The model under review builds one solid part; all positions refer to its coordinate system, in mm. A direction names the side the tool comes from. Round coordinates to 2 decimals unless told otherwise and drop trailing zeros. Loops run counter-clockwise (first coordinate to the right, second up) from the corner with the lowest first, then second, coordinate; pieces in that order, holes last. Notation, with made-up numbers: M -11.75,38 L 27.25,38 A25 cw 27.25,52 Z; hole C -15,21.5 d5. An arc over 180 degrees is marked long. One line per question, with ' | ' between items.
Autodesk Inventor part; units mm, degrees
ref_plane "YZ Plane" through (0, 0, 0) normal (1, 0, 0) x (0, 1, 0)
ref_plane "XZ Plane" through (0, 0, 0) normal (0, 1, 0) x (-1, 0, 0)
ref_plane "XY Plane" through (0, 0, 0) normal (0, 0, 1) x (1, 0, 0)
sketch "スケッチ1" plane through (0, 0, 0) normal (0, 0, 1) x (1, 0, 0)
  line L0 (51, 14.4226) -> (51, -10.5774)
  line L1 (-51, -10.5774) -> (-51, 14.4226)
  circle A0 centre (-22.5, -0.0774) radius 1.6
  circle A1 centre (22.5, -0.0774) radius 1.6
  line L2 (-71, -27.5774) -> (71, -27.5774)
  line L3 (71, -27.5774) -> (71, -14.5774)
  line L4 (-53, -12.5774) -> (-69, -12.5774)
  line L5 (-71, -14.5774) -> (-71, -27.5774)
  arc A2 (-53, -12.5774) -> (-51, -10.5774) centre (-53, -10.5774) ccw
  line L6 (69, -12.5774) -> (53, -12.5774)
  arc A3 (51, -10.5774) -> (53, -12.5774) centre (53, -10.5774) ccw
  line L7 (-51, 14.4226) -> (51, 14.4226)
  arc A4 (-69, -12.5774) -> (-71, -14.5774) centre (-69, -14.5774) ccw
  arc A5 (71, -14.5774) -> (69, -12.5774) centre (69, -14.5774) ccw
  arc A6 (51, 14.4226) -> (-51, 14.4226) centre (0, -53.5774) ccw
  point P0 (0, 0)
  point P1 (0, -100)
  point P2 (71, -12.5774)
  point P3 (-71, -12.5774)
  point P4 (0, 31.4226)
  dimension "d5" = 51
  dimension "d8" = 3.2
  dimension "d10" = 3.2
  dimension "d28" = 45
  dimension "d31" = 28.5
  dimension "d35" = 142
  dimension "d36" = 15
  dimension "d38" = 2
  dimension "d39" = 2
  dimension "d42" = 20
  dimension "d47" = 100
  dimension "d48" = 51
  dimension "d55" = 102
  dimension "d56" = 42
  dimension "d57" = 2
  dimension "d58" = 2
  dimension "d73" = 27.5
  dimension "d75" = 27.5
  dimension "d76" = 17
  dimension "d86" = 20
extrude "押し出し1" add sketch "スケッチ1" along normal blind 38
sketch "スケッチ2" plane through (0, 0, 38) normal (0, 0, 1) x (1, 0, 0)
  line L0 (-39, 13.4226) -> (39, 13.4226)
  line L1 (46, 6.4226) -> (46, -10.5774)
  line L2 (44, -12.5774) -> (-44, -12.5774)
  line L3 (-46, -10.5774) -> (-46, 6.4226)
  arc A0 (-39, 13.4226) -> (-46, 6.4226) centre (-39, 6.4226) ccw
  arc A1 (46, 6.4226) -> (39, 13.4226) centre (39, 6.4226) ccw
  arc A2 (-46, -10.5774) -> (-44, -12.5774) centre (-44, -10.5774) ccw
  arc A3 (44, -12.5774) -> (46, -10.5774) centre (44, -10.5774) ccw
  circle A4 centre (22.5, -0.0774) radius 1.6
  point P0 (0, 0)
  point P1 (-46, 13.4226)
  point P2 (46, -12.5774)
  point P3 (46, 13.4226)
  point P4 (-46, -12.5774)
  dimension "d17" = 92
  dimension "d18" = 26
  dimension "d19" = 46
  dimension "d23" = 7
  dimension "d24" = 7
  dimension "d25" = 2
  dimension "d26" = 2
  dimension "d50" = 12.5
extrude "押し出し2" cut sketch "スケッチ2" against normal blind 33 contours L0 A1 L1 A3 L2 A2 L3 A0 | A4
sketch "スケッチ3" plane through (0, 0, 38) normal (0, 0, 1) x (1, 0, 0)
  line L0 (-39, 13.4226) -> (39, 13.4226)
  arc A0 (39, 13.4226) -> (-39, 13.4226) centre (0, -57.6274) ccw
  line L1 (-46, -10.5774) -> (-46, 6.4226)
  line L2 (44, -12.5774) -> (-44, -12.5774)
  line L3 (-39, 13.4226) -> (39, 13.4226)
  point P0 (0, 0)
  point P1 (0, 23.4226)
  dimension "d59" = 10
extrude "押し出し3" cut sketch "スケッチ3" against normal blind 40
sketch "スケッチ4" plane through (0, 0, 38) normal (0, 0, 1) x (1, 0, 0)
  line L0 (-31, -12.5774) -> (31, -12.5774)
  line L1 (31, -12.5774) -> (31, -20.5774)
  line L2 (29, -22.5774) -> (-29, -22.5774)
  line L3 (-31, -20.5774) -> (-31, -12.5774)
  line L4 (-46, -10.5774) -> (-46, 6.4226)
  line L5 (44, -12.5774) -> (-44, -12.5774)
  arc A0 (-31, -20.5774) -> (-29, -22.5774) centre (-29, -20.5774) ccw
  arc A1 (29, -22.5774) -> (31, -20.5774) centre (29, -20.5774) ccw
  point P0 (0, 0)
  point P1 (31, -22.5774)
  point P2 (-31, -22.5774)
  dimension "d66" = 62
  dimension "d67" = 10
  dimension "d68" = 15
  dimension "d69" = 10
  dimension "d72" = 2
extrude "押し出し4" cut sketch "スケッチ4" against normal blind 35
sketch "スケッチ5" plane through (-69, -12.5774, 0) normal (0, 1, 0) x (1, 0, 0)
  circle A0 centre (8, -18) radius 5.05
  line L0 (69, 0) -> (69, -40)
  circle A1 centre (130, -18) radius 5.05
  line L1 (18, 0) -> (18, -38)
  line L2 (16, -38) -> (0, -38)
  point P0 (-2, -38)
  dimension "d77" = 10.1
  dimension "d84" = 10
  dimension "d85" = 20
extrude "押し出し5" cut sketch "スケッチ5" against normal blind 5
sketch "スケッチ6" plane through (-61, -17.5774, 18) normal (0, 1, 0) x (1, 0, 0)
  line L0 (61, 18) -> (61, -20)
  line L1 (90, -20) -> (32, -20)
  circle A0 centre (0, 0) radius 2.6
  circle A1 centre (122, 0) radius 2.6
  line L2 (10, 18) -> (10, -20)
  line L3 (8, -20) -> (-8, -20)
  dimension "d81" = 5.2
  dimension "d87" = 10
  dimension "d88" = 20
extrude "押し出し6" cut sketch "スケッチ6" against normal blind 10
sketch "スケッチ7" plane through (-51, -10.5774, 0) normal (-1, 0, 0) x (0, 0, 1)
  line L0 (7, 19) -> (11, 19)
  line L1 (13, 17) -> (13, 5)
  line L2 (11, 3) -> (7, 3)
  line L3 (5, 5) -> (5, 17)
  arc A0 (7, 19) -> (5, 17) centre (7, 17) ccw
  arc A1 (5, 5) -> (7, 3) centre (7, 5) ccw
  arc A2 (11, 3) -> (13, 5) centre (11, 5) ccw
  arc A3 (13, 17) -> (11, 19) centre (11, 17) ccw
  line L4 (0, 25) -> (0, 0)
  point P0 (0, 10.5774)
  point P1 (13, 3)
  point P2 (13, 19)
  point P3 (5, 3)
  point P4 (38, -2)
  dimension "d89" = 8
  dimension "d90" = 16
  dimension "d91" = 2
  dimension "d94" = 5
  dimension "d95" = 5
extrude "押し出し7" cut sketch "スケッチ7" against normal blind 8
properties part number "jig"
1) For line 1 (Z direction, x = -61, y = -16); line 2 (Z direction, x = -46.5, y = 5); line 3 (X direction, y = -22.25, z = 18), list the stretches that pass through material, from the lowest coordinate up.
Output values:
line 1: z = 0 to 12.95, 23.05 to 38 | line 2: z = 0 to 5, 13 to 38 | line 3: x = -71 to -63.6, -58.4 to -30.1, 30.1 to 58.4, 63.6 to 71
2) Machinability: for faces 1 (the flat face through (-59, -12.577, 23)), 2 (the flat face through (0, -22.577, 21)), 3 (the flat face through (-1, -27.577, 19)), 4 (the flat face through (-59, -17.577, 20)), which of the approach directions +Z, -Z, +X, -X, +Y, -Y give a long, thin tool a straight path to every point of the face, cutting with its end or side? Answer none if there is none.
Output values:
face 1: +Z, -Z, -X, +Y | face 2: +Z | face 3: +Z, -Z, +X, -X, -Y | face 4: +Y
3) Add section B-B on z = 31. State the section outline as (x, y) points, then the cut area to 3 significant figures.
Output values:
outline: M -71,-27.58 L 71,-27.58 L 71,-14.58 A2 ccw 69,-12.58 L 53,-12.58 A2 cw 51,-10.58 L 51,14.42 A85 ccw -51,14.42 L -51,-10.58 A2 cw -53,-12.58 L -69,-12.58 A2 ccw -71,-14.58 Z; hole M -46,-10.58 A2 ccw -44,-12.58 L -31,-12.58 L -31,-20.58 A2 ccw -29,-22.58 L 29,-22.58 A2 ccw 31,-20.58 L 31,-12.58 L 44,-12.58 A2 ccw 46,-10.58 L 46,6.42 A7 ccw 39,13.42 A81.05 ccw -39,13.42 A7 ccw -46,6.42 Z | area: 2,550 mm²
4) Add section D-D on x = -22.5. State the section outline as (y, z) points, then the cut area to 3 significant figures.
Output values:
outline: M -27.58,0 L -1.68,0 L -1.68,5 L -12.58,5 L -12.58,3 L -22.58,3 L -22.58,38 L -27.58,38 Z; M 1.52,0 L 13.42,0 L 13.42,5 L 1.52,5 Z; M 20.24,0 L 28.39,0 L 28.39,38 L 20.24,38 Z | area: 644 mm²
5) Mouldability with a two-part tool opening along Y and no side actions: class faces 5 (the flat face through (63, -12.577, 23)), 6 (the flat face through (-37, -12.577, 22)), 7 (the cylindrical face through (-43.895, 11.426, 21.731)), 8 (the flat face through (-51, 2, 19)) as +Y half, -Y half, draft (parallel to the pull), parting line (faces both ways), or undercut.
Output values:
face 5: +Y half | face 6: undercut | face 7: undercut | face 8: draft
6) Add section A-A on x = -61. State the section outline as (y, z) points.
Output values:
outline: M -27.58,0 L -12.58,0 L -12.58,12.95 L -17.58,12.95 L -17.58,15.4 L -27.58,15.4 Z; M -27.58,20.6 L -17.58,20.6 L -17.58,23.05 L -12.58,23.05 L -12.58,38 L -27.58,38 Z
7) Add section C-C on y = -4. State the section outline as (x, z) points, then the cut area to 3 significant figures.
Output values:
outline: M -51,0 L 51,0 L 51,38 L 46,38 L 46,5 L -51,5 Z; M -51,13 L -46,13 L -46,38 L -51,38 Z | area: 800 mm²
8) Insertion check: P1, Ø1.5, axis at x = -49, y = -1, coming from the -Z side; P2, Ø8.5, axis at x = 61, z = 18, coming from the +Y side; P3, Ø5, axis at x = -63, z = 20, coming from the +Y side; P4, Ø4, axis at x = 39.5, z = 23, coming from the +Y side. Each pin has a flat end and moves straight along its axis. Give the tip position at first contact, or say it passes through.
Output values:
P1: stops at z = 0 | P2: stops at y = -17.58 | P3: stops at y = -12.58 | P4: stops at y = 22.7
